For this review, take the finished solid that the model builds, in its own axes (mm). Give positions to 0.01 mm unless a question says otherwise; leave off trailing zeros. Write each loop counter-clockwise with the first axis right and the second up, starting at its lowest first coordinate (ties: lowest second). Pieces come first, ordered by that corner, then holes. Notation, with made-up numbers: (-1, 5.25) -> (50, 5.25) arc R29 ccw to (50, 27.25) -> close; hole circle Ø6 at (49, -8.75). An arc over 180 degrees is marked (long way). Answer as CSV lines item,"result".
```python
from build123d import *

# Parameters (mm, degrees)
SKETCH_1_R           = 1.55
EXTRUDE_1_DEPTH      = 2.5
FILLET_1_R           = 1
CHAMFER_1_SIZE       = 3
SKETCH_3_R           = 2.05
CUT_EXTRUDE_1_DEPTH  = 178.05212527
CUT_EXTRUDE_2_DEPTH  = 178.05212527
CUT_EXTRUDE_3_DEPTH  = 166.292604008
FILLET_2_R           = 1
CHAMFER_2_SIZE       = 4.5
FILLET_4_R           = 5
EXTRUDE_3_DEPTH      = 5
FILLET_5_R           = 1
FILLET_7_R           = 1
CUT_EXTRUDE_4_DEPTH  = 165.600736622
FILLET_8_R           = 1
CUT_EXTRUDE_5_DEPTH  = 165.600736622
EXTRUDE_5_DEPTH      = 5
CUT_EXTRUDE_6_DEPTH  = 165.600736622
FILLET_9_R           = 1
CUT_EXTRUDE_7_DEPTH  = 165.600736622
SKETCH_13_R          = 4.5
SKETCH_13_R_2        = 2.05
EXTRUDE_6_DEPTH      = 5
FILLET_10_R          = 1
EXTRUDE_7_DEPTH      = 5
FILLET_11_R          = 1
EXTRUDE_8_DEPTH      = 5
SKETCH_17_R          = 1
CUT_EXTRUDE_9_DEPTH  = 165.600736622
CHAMFER_3_SIZE       = 1
SKETCH_18_R          = 2.05
CUT_EXTRUDE_10_DEPTH = 165.600736622


with BuildPart() as part:
    # 草图1 → 凸台-拉伸1 (new, symmetric)
    with BuildSketch(Plane.XY):
        with BuildLine():
            Line((-6, -14.025), (-14, -14.025))
            Line((-14, -14.025), (-14, -29.025))
            Line((-14, -29.025), (171.107064417, -45.219769675))
            Line((171.107064417, -45.219769675), (152.100622615, 7))
            Line((152.100622615, 7), (141.5, 7))
            Line((141.5, 7), (141.5, -14.025))
            Line((141.5, -14.025), (8.5, -14.025))
            Line((8.5, -14.025), (8.5, 7))
            Line((8.5, 7), (-8.5, 7))
            Line((-8.5, 7), (-8.5, -8.975))
            Line((-8.5, -8.975), (-6, -8.975))
            ThreePointArc((-6, -8.975), (-3.475, -11.5), (-6, -14.025))
        make_face()
        with Locations((-5, 3.5)):
            Circle(SKETCH_1_R, mode=Mode.SUBTRACT)
        with Locations((5, 3.5)):
            Circle(SKETCH_1_R, mode=Mode.SUBTRACT)
        with Locations((-5, -3.5)):
            Circle(SKETCH_1_R, mode=Mode.SUBTRACT)
        with Locations((5, -3.5)):
            Circle(SKETCH_1_R, mode=Mode.SUBTRACT)
        with Locations((145, 3.5)):
            Circle(SKETCH_1_R, mode=Mode.SUBTRACT)
        with Locations((145, -3.5)):
            Circle(SKETCH_1_R, mode=Mode.SUBTRACT)
        Polygon((148, 4), (148, -13.5), (156.3694791, -13.5), (150, 4), align=None, mode=Mode.SUBTRACT)
    extrude(amount=EXTRUDE_1_DEPTH, both=True)

    # 圆角1
    fillet_1_edges = [part.edges().sort_by_distance(p)[0] for p in [
        (141.5, 7, 0),
        (152.100622615, 7, 0),
        (156.3694791, -13.5, 0),
        (150, 4, 0),
        (148, 4, 0),
        (148, -13.5, 0),
    ]]
    fillet(fillet_1_edges, radius=FILLET_1_R)

    # 倒角1
    chamfer_1_edges = [part.edges().sort_by_distance(p)[0] for p in [
        (8.5, -14.025, 0),
        (141.5, -14.025, 0),
    ]]
    chamfer(chamfer_1_edges, length=CHAMFER_1_SIZE)

    # 草图3 → 切除-拉伸1 (cut, through all)
    with BuildSketch(Plane.XY.offset(2.5)):
        with Locations((-9, -24.5)):
            Circle(SKETCH_3_R)
        with Locations((146, -21.5)):
            Circle(SKETCH_3_R)
        with Locations((134, -36.5)):
            Circle(SKETCH_3_R)
    extrude(amount=-CUT_EXTRUDE_1_DEPTH, mode=Mode.SUBTRACT)

    # 草图4 → 切除-拉伸2 (cut, through all)
    with BuildSketch(Plane.XY.offset(2.5)):
        Polygon((159.725158013, -13.94823884), (137.088896577, -42.243565635), (171.107064417, -45.219769675), align=None)
    extrude(amount=-CUT_EXTRUDE_2_DEPTH, mode=Mode.SUBTRACT)

    # 草图5 → 切除-拉伸3 (cut, through all)
    with BuildSketch(Plane.XY.offset(2.5)):
        with BuildLine():
            Line((-12.181980515, -21.318019485), (-8.888961031, -18.025))
            Line((-8.888961031, -18.025), (143.140913607, -18.025))
            ThreePointArc((143.140913607, -18.025), (141.625936704, -22.557151967), (145.043511375, -25.8971729))
            Line((145.043511375, -25.8971729), (138.079963863, -34.60160729))
            ThreePointArc((138.079963863, -34.60160729), (132.505892934, -32.255280448), (129.630475707, -37.575759011))
            Line((129.630475707, -37.575759011), (-4.699014499, -25.823451441))
            ThreePointArc((-4.699014499, -25.823451441), (-6.678842462, -20.644844013), (-12.181980515, -21.318019485))
        make_face()
    extrude(amount=-CUT_EXTRUDE_3_DEPTH, mode=Mode.SUBTRACT)

    # 圆角2
    fillet_2_edges = [part.edges().sort_by_distance(p)[0] for p in [
        (-4.699014499, -25.823451441, 0),
        (-8.888961031, -18.025, 0),
        (143.140913607, -18.025, 0),
        (145.043511375, -25.8971729, 0),
        (138.079963863, -34.60160729, 0),
        (129.630475707, -37.575759011, 0),
    ]]
    fillet(fillet_2_edges, radius=FILLET_2_R)
    fillet_2_2_edges = [part.edges().sort_by_distance(p)[0] for p in [
        (-12.181980515, -21.318019485, 0),
    ]]
    fillet(fillet_2_2_edges, radius=FILLET_2_R)

    # 倒角2
    chamfer_2_edges = [part.edges().sort_by_distance(p)[0] for p in [
        (-14, -14.025, 0),
    ]]
    chamfer(chamfer_2_edges, length=CHAMFER_2_SIZE)

    # 圆角4
    fillet_4_edges = [part.edges().sort_by_distance(p)[0] for p in [
        (159.725158013, -13.94823884, 0),
        (137.088896577, -42.243565635, 0),
        (-14, -29.025, 0),
    ]]
    fillet(fillet_4_edges, radius=FILLET_4_R)

    # 草图7 → 凸台-拉伸3 (add)
    with BuildSketch(Plane.XY.offset(2.5)):
        Polygon((16.525252532, -18.025), (46.483701437, -30.301358854), (59.896469489, -31.474824005), (27.074370524, -18.025), align=None)
        Polygon((102.074370524, -18.025), (74.83938996, -32.782160146), (82.068385362, -33.414615292), (110.470589391, -18.025), align=None)
    extrude(amount=-EXTRUDE_3_DEPTH)

    # 圆角5
    fillet_5_edges = [part.edges().sort_by_distance(p)[0] for p in [
        (16.525252532, -18.025, 0),
        (27.074370524, -18.025, 0),
        (59.896469489, -31.474824005, 0),
        (46.483701437, -30.301358854, 0),
        (102.074370524, -18.025, 0),
        (110.470589391, -18.025, 0),
        (82.068385362, -33.414615292, 0),
        (74.83938996, -32.782160146, 0),
    ]]
    fillet(fillet_5_edges, radius=FILLET_5_R)

    # 圆角7
    fillet_7_edges = [part.edges().sort_by_distance(p)[0] for p in [
        (-8.5, 7, 0),
        (8.5, 7, 0),
    ]]
    fillet(fillet_7_edges, radius=FILLET_7_R)

    # 草图8 → 切除-拉伸4 (cut, through all)
    with BuildSketch(Plane.XY.offset(2.5)):
        with BuildLine():
            Line((1.732359313, -8.5), (7.257359313, -14.025))
            Line((7.257359313, -14.025), (-1.08573505, -14.025))
            ThreePointArc((-1.08573505, -14.025), (-0.481816001, -11.225645569), (-1.36042836, -8.5))
            Line((-1.36042836, -8.5), (1.732359313, -8.5))
        make_face()
    extrude(amount=-CUT_EXTRUDE_4_DEPTH, mode=Mode.SUBTRACT)

    # 圆角8
    fillet_8_edges = [part.edges().sort_by_distance(p)[0] for p in [
        (-1.36042836, -8.5, 0),
        (1.732359313, -8.5, 0),
        (7.257359313, -14.025, 0),
        (-1.08573505, -14.025, 0),
    ]]
    fillet(fillet_8_edges, radius=FILLET_8_R)

    # 草图9 → 切除-拉伸5 (cut, through all)
    with BuildSketch(Plane.XY.offset(2.5)):
        Polygon((8.5, -11.025), (7.085786438, -9.610786438), (8.5, -8.196572875), align=None)
    extrude(amount=-CUT_EXTRUDE_5_DEPTH, mode=Mode.SUBTRACT)

    # 草图10 → 凸台-拉伸5 (add)
    with BuildSketch(Plane.XY.offset(2.5)):
        Polygon((8.5, -8.196572875), (14.328427125, -14.025), (18.571067812, -14.025), (8.5, -3.953932188), align=None)
    extrude(amount=-EXTRUDE_5_DEPTH)

    # 草图11 → 切除-拉伸6 (cut, through all)
    with BuildSketch(Plane.XY.offset(2.5)):
        with BuildLine():
            Line((-4.214555378, -9.714555378), (-8.5, -5.429110755))
            Line((-8.5, -5.429110755), (-8.5, -8.975))
            Line((-8.5, -8.975), (-6, -8.975))
            ThreePointArc((-6, -8.975), (-5.033724333, -9.16720418), (-4.214555378, -9.714555378))
        make_face()
    extrude(amount=-CUT_EXTRUDE_6_DEPTH, mode=Mode.SUBTRACT)

    # 圆角9
    fillet_9_edges = [part.edges().sort_by_distance(p)[0] for p in [
        (8.5, -3.953932188, 0),
        (18.571067812, -14.025, 0),
        (14.328427125, -14.025, 0),
        (11.5, -14.025, 0),
        (138.5, -14.025, 0),
        (7.085786438, -9.610786438, 0),
        (8.5, -8.196572875, 0),
        (-8.5, -5.429110755, 0),
        (141.5, -11.025, 0),
    ]]
    fillet(fillet_9_edges, radius=FILLET_9_R - 0.0001)  # a hair under: the kernel refuses the full size

    # 草图12 → 切除-拉伸7 (cut, through all)
    with BuildSketch(Plane.XY.offset(2.5)):
        with BuildLine():
            Line((-3, 7), (-1.5, 5))
            Line((-1.5, 5), (-1.5, -1))
            ThreePointArc((-1.5, -1), (0, -2.5), (1.5, -1))
            Line((1.5, -1), (1.5, 5))
            Line((1.5, 5), (3, 7))
            Line((3, 7), (-3, 7))
        make_face()
    extrude(amount=-CUT_EXTRUDE_7_DEPTH, mode=Mode.SUBTRACT)

    # 草图13 → 凸台-拉伸6 (add)
    with BuildSketch(Plane.XY.offset(2.5)):
        with Locations((111, -19.5)):
            Circle(SKETCH_13_R)
        with Locations((111, -19.5)):
            Circle(SKETCH_13_R_2, mode=Mode.SUBTRACT)
    extrude(amount=-EXTRUDE_6_DEPTH)

    # 圆角10
    fillet_10_edges = [part.edges().sort_by_distance(p)[0] for p in [
        (106.547310536, -20.150812215, 0),
    ]]
    fillet(fillet_10_edges, radius=FILLET_10_R)

    # 草图15 → 凸台-拉伸7 (add)
    with BuildSketch(Plane.XY.offset(2.5)):
        with BuildLine():
            Line((113.052955542, -23.504419252), (129.569480214, -35.712285314))
            ThreePointArc((129.569480214, -35.712285314), (130.381207363, -33.825240225), (131.947044458, -32.495580748))
            Line((131.947044458, -32.495580748), (115.430519786, -20.287714686))
            ThreePointArc((115.430519786, -20.287714686), (114.618792637, -22.174759775), (113.052955542, -23.504419252))
        make_face()
    extrude(amount=-EXTRUDE_7_DEPTH)

    # 圆角11
    fillet_11_edges = [part.edges().sort_by_distance(p)[0] for p in [
        (115.251396829, -18.025, 0),
        (113.052955542, -23.504419252, 0),
        (115.430519786, -20.287714686, 0),
        (131.947044458, -32.495580748, 0),
        (129.569480214, -35.712285314, 0),
    ]]
    fillet(fillet_11_edges, radius=FILLET_11_R)

    # 草图16 → 凸台-拉伸8 (add)
    with BuildSketch(Plane.XY.offset(2.5)):
        with BuildLine():
            Line((7.5, 7), (18, 7))
            Line((18, 7), (18, 0.5))
            Line((18, 0.5), (8.5, 0.5))
            Line((8.5, 0.5), (8.5, 6))
            ThreePointArc((8.5, 6), (8.207106781, 6.707106781), (7.5, 7))
        make_face()
    extrude(amount=-EXTRUDE_8_DEPTH)

    # 草图17 → 切除-拉伸9 (cut, through all)
    with BuildSketch(Plane.XY.offset(2.5)):
        with Locations((9.5, 0.5)):
            Circle(SKETCH_17_R)
        with Locations((9.5, 7)):
            Circle(SKETCH_17_R)
    extrude(amount=-CUT_EXTRUDE_9_DEPTH, mode=Mode.SUBTRACT)

    # 倒角3
    chamfer_3_edges = [part.edges().sort_by_distance(p)[0] for p in [
        (18, 7, 0),
        (18, 0.5, 0),
    ]]
    chamfer(chamfer_3_edges, length=CHAMFER_3_SIZE)

    # 草图18 → 切除-拉伸10 (cut, through all)
    with BuildSketch(Plane.XY.offset(2.5)):
        with Locations((111, -19.5)):
            Circle(SKETCH_18_R)
    extrude(amount=-CUT_EXTRUDE_10_DEPTH, mode=Mode.SUBTRACT)


solid = part.part
```
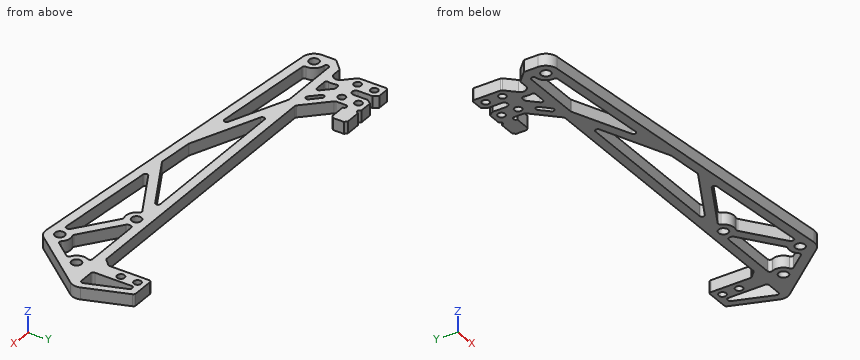
Q1. To check wall thickness, follow probe 1 along X at (y, z) = (-12, 0.7) (3 decimals); probe 2 along Y at (x, z) = (11, -2.05) (3 decimals); probe 3 along Y at (x, z) = (-5, 0.3) (3 decimals). State the ranges of each line that lie inside material, in increasing order. Write a range as [from, to].
Answer block:
probe 1,"x = [-3.525, -0.498], [5.232, 9.475], [12.303, 16.546], [140.525, 148], [155.824, 158.961]"
probe 2,"y = [-31.212, -27.197], [-18.025, -13.525], [-10.697, -6.454], [0.5, 7]"
probe 3,"y = [-29.812, -22.438], [-18.025, -13.819], [-8.929, -5.05], [-1.95, 1.95], [5.05, 7]"
Q2. Add section B-B (z = -1.6). State how many separate pieces and enclosed holes the cut face has, plus the area to 3 significant figures.
Answer block:
separate pieces,"1"
enclosed holes,"17"
area,"2,420 mm2"
Q3. Add section A-A (x = 54). Write out the cut boundary in (y, z) (3 decimals), plus the area to 3 significant figures.
Answer block:
outline,"(-34.974, -2.5) -> (-29.059, -2.5) -> (-29.059, 2.5) -> (-34.974, 2.5) -> close; (-18.025, -2.5) -> (-14.025, -2.5) -> (-14.025, 2.5) -> (-18.025, 2.5) -> close"
area,"49.6 mm2"
Q4. Clearance check with flat-ended pins moving along their axes: pin 1 (1.5 mm diameter, centred on y = -2, z = 0, fed in from -X); pin 2 (1.5 mm diameter, centred on x = 66, z = 0, fed in from -Y); pin 3 (3 mm diameter, centred on y = -0.5, z = -0.5, fed in from +X). State where each tip first meets the part, or that it passes through.
Answer block:
pin 1,"stops at x = -8.5"
pin 2,"stops at y = -36.09"
pin 3,"stops at x = 155.38"
